Check sheet for the modelled part. Datum: model origin and axes. Units: mm. Face numbers are marked on the shaded views. Round coordinates to 2 decimals unless told otherwise and drop trailing zeros. Order: outer loops, then holes, each group sorted by start corner. A loop starts at its lowest first (then second) coordinate and runs counter-clockwise, first axis right, second up.
Q1. Scan lines: probe 1 along Z at (x, y) = (-32.5, -4); probe 2 along X at (y, z) = (-3.8, 11); probe 3 along Y at (x, z) = (20, -21). Record each from-to range of solid material in increasing order.
Q2. Mould release check, pull along X, two halves, no side actions. Record for the marked faces 1 and 2: +X half, -X half, draft (parallel to the pull), parting line (faces both ways), or undercut.
Q3. Cross-section at B-B on x = -16. Record the cut outline in (y, z), then the cut area to 4 significant figures.
Q4. Cross-section at C-C on z = 5. Record the cut outline in (x, y), then the cut area to 3 significant figures.
Q5. Depth check by flat-ended pin: P1, Ø5, axis at x = 49.5, z = 22.5, coming from the +Y side; P2, Ø1.5, axis at x = 23, z = 2.5, coming from the -Y side; P3, Ø0.5, axis at x = 57.5, y = -4, coming from the +Z side; P4, Ø0.6, axis at y = -4.5, z = -52, coming from the +X side. Enter the tip coordinate at first touch or a pass-through.
Q6. Cross-section at A-A on y = -4.5. Record the cut outline in (x, z).
from build123d import *

# Parameters (mm, degrees)
F0_W      = 120
F0_H      = 101
F1_DEPTH  = 4
F0_W_2    = 124
F0_H_2    = 105
F2_DEPTH  = 5
F3_DEPTH  = 0.5
F4_R      = 5
F5_R      = 2
F6_W      = 2
F6_H      = 2
F7_DEPTH  = 1.5
F8_W      = 2
F8_H      = 2
F9_DEPTH  = 1.5
F10_DEPTH = 0.5


with BuildPart() as f1:
    # F0 (on Front) → F1 (new body)
    with BuildSketch(Plane.XZ):
        Rectangle(F0_W, F0_H)
    extrude(amount=F1_DEPTH)

    # F0 (on Front) → F2 (join)
    with BuildSketch(Plane.XZ):
        Rectangle(F0_W_2, F0_H_2)
        Rectangle(F0_W, F0_H, mode=Mode.SUBTRACT)
    extrude(amount=F2_DEPTH)

    # F3 (add): a face of the model
    f3_faces = [f1.faces().sort_by_distance(p)[0] for p in [
        (0, -5, -50.8751615465),
    ]]
    extrude(f3_faces, amount=F3_DEPTH)

    # F4
    f4_edges = [f1.edges().sort_by_distance(p)[0] for p in [
        (62, -2.75, -52.5),
        (-62, -2.75, -52.5),
        (-62, -2.75, 52.5),
        (62, -2.75, 52.5),
    ]]
    fillet(f4_edges, radius=F4_R)

    # F5
    f5_edges = [f1.edges().sort_by_distance(p)[0] for p in [
        (60, -4.75, 50.5),
        (-60, -4.75, -50.5),
        (60, -4.75, -50.5),
        (-60, -4.75, 50.5),
    ]]
    fillet(f5_edges, radius=F5_R)

    # F6 (on face) → F7 (cut)
    with BuildSketch(Plane.XZ.offset(5.5)):
        with Locations((-56, -51.5)):
            Rectangle(F6_W, F6_H)
    extrude(amount=-F7_DEPTH, mode=Mode.SUBTRACT)

    # F8 (on face) → F9 (cut)
    with BuildSketch(Plane.XZ.offset(5.5)):
        with Locations((56, -51.5)):
            Rectangle(F8_W, F8_H)
    extrude(amount=-F9_DEPTH, mode=Mode.SUBTRACT)

    # F10 (cut): a face of the model
    f10_faces = [f1.faces().sort_by_distance(p)[0] for p in [
        (0, -4, -0.0339805967),
    ]]
    extrude(f10_faces, amount=-F10_DEPTH, mode=Mode.SUBTRACT)


solid = f1.part
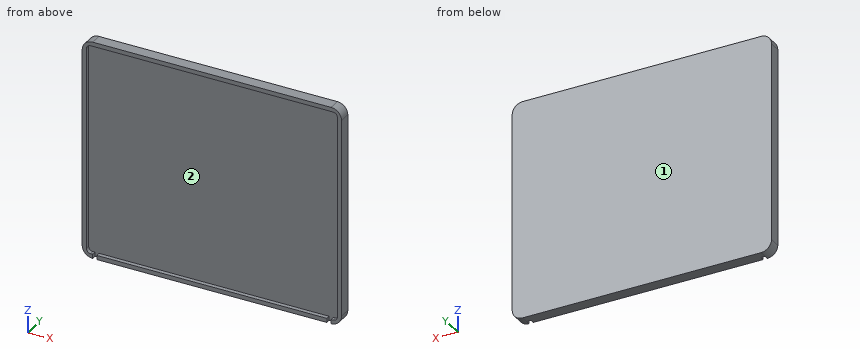
Results found:
1. probe 1: z = -52.5 to -50.5, 50.5 to 52.5
1. probe 2: x = -62 to -60, 60 to 62
1. probe 3: y = -3.5 to 0
2. face 1: draft
2. face 2: undercut
3. outline: (-5.5, -52.5) - (0, -52.5) - (0, 52.5) - (-5.5, 52.5) - (-5.5, 50.5) - (-3.5, 50.5) - (-3.5, -50.5) - (-5.5, -50.5) - close
3. area: 375.5 mm2
4. outline: (-62, -5.5) - (-60, -5.5) - (-60, -3.5) - (60, -3.5) - (60, -5.5) - (62, -5.5) - (62, 0) - (-62, 0) - close
4. area: 442 mm2
5. P1: stops at y = 0
5. P2: stops at y = -3.5
5. P3: stops at z = 52.49
5. P4: stops at x = 59.71
6. outline: (-62, -47.5) arc R5 ccw to (-57, -52.5) - (-57, -50.5) - (-58, -50.5) arc R2 cw to (-60, -48.5) - (-60, 48.5) arc R2 cw to (-58, 50.5) - (58, 50.5) arc R2 cw to (60, 48.5) - (60, -48.5) arc R2 cw to (58, -50.5) - (57, -50.5) - (57, -52.5) arc R5 ccw to (62, -47.5) - (62, 47.5) arc R5 ccw to (57, 52.5) - (-57, 52.5) arc R5 ccw to (-62, 47.5) - close; (-55, -52.5) - (55, -52.5) - (55, -50.5) - (-55, -50.5) - close
